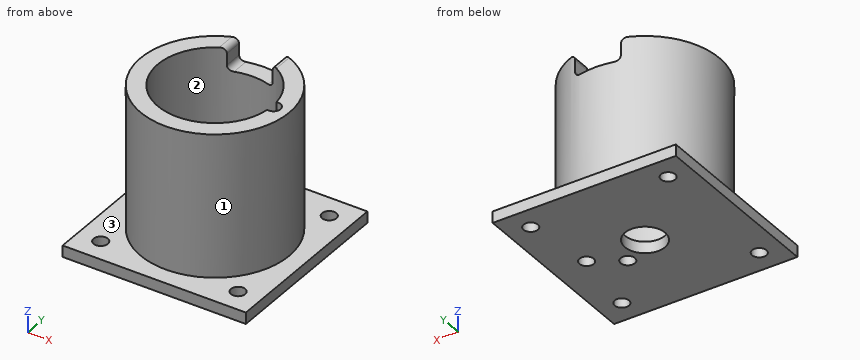
Autodesk Inventor part; units mm, degrees
ref_plane "Work Plane1" through (0, 16.51, 0) normal (0, 1, 0) x (-1, 0, 0)
ref_plane "YZ Plane" through (0, 0, 0) normal (1, 0, 0) x (0, 1, 0)
ref_plane "XY Plane" through (0, 0, 0) normal (0, 0, 1) x (1, 0, 0)
sketch "Sketch1" plane through (0, 0, 0) normal (0, 0, 1) x (1, 0, 0)
  line L0 (20.32, 20.32) -> (-20.32, 20.32)
  line L1 (-20.32, 20.32) -> (-20.32, -20.32)
  line L2 (-20.32, -20.32) -> (20.32, -20.32)
  line L3 (20.32, -20.32) -> (20.32, 20.32)
  point P0 (0, 0)
  dimension "d0" = 40.64
  dimension "d1" = 40.64
  dimension "d2" = 20.32
  dimension "d3" = 20.32
extrude "Extrusion1" add sketch "Sketch1" along normal blind 2.54
sketch "Sketch2" plane through (0, 0, 2.54) normal (0, 0, 1) x (1, 0, 0)
  circle A0 centre (0, 0) radius 12.7
  circle A1 centre (0, 0) radius 16.51
  dimension "d6" = 25.4
  dimension "d7" = 3.81
extrude "Extrusion2" add sketch "Sketch2" along normal blind 31.75
sketch "Sketch3" plane through (0, 0, 2.54) normal (0, 0, 1) x (1, 0, 0)
  line L0 (20.32, 20.32) -> (-20.32, 20.32)
  line L1 (-20.32, 20.32) -> (-20.32, -20.32)
  line L2 (20.32, -20.32) -> (20.32, 20.32)
  line L3 (-20.32, -20.32) -> (20.32, -20.32)
  point P0 (0, 0)
  point P1 (-15.24, -15.24)
  point P2 (15.24, -15.24)
  point P3 (15.24, 15.24)
  point P4 (-15.24, 15.24)
  dimension "d10" = 5.08
  dimension "d11" = 5.08
  dimension "d12" = 5.08
  dimension "d13" = 5.08
  dimension "d14" = 5.08
  dimension "d15" = 5.08
  dimension "d16" = 5.08
  dimension "d17" = 5.08
hole "Hole1" at (-15.24, -15.24, 2.54) at (15.24, -15.24, 2.54) at (15.24, 15.24, 2.54) at (-15.24, 15.24, 2.54) direction (0, 0, -1) diameter 3.175 depth 3.175 tip angle 118
ref_plane "Work Plane1" through (0, 16.51, 0) normal (0, 1, 0) x (-1, 0, 0)
sketch "Sketch4" plane through (0, 16.51, 0) normal (0, 1, 0) x (-1, 0, 0)
  line L0 (-12.7, 34.29) -> (12.7, 34.29)
  line L1 (5.08, 34.29) -> (-5.08, 34.29)
  line L2 (-5.08, 34.29) -> (-5.08, 29.21)
  line L3 (-5.08, 29.21) -> (5.08, 29.21)
  line L4 (5.08, 29.21) -> (5.08, 34.29)
  line L5 (0, -6.858) -> (0, 41.148)
  point P0 (0, 0)
  dimension "d26" = 5.08
  dimension "d27" = 10.16
  dimension "d28" = 5.08
extrude "Extrusion3" cut sketch "Sketch4" against normal blind 10.16
sketch "Sketch5" plane through (0, 0, 2.54) normal (0, 0, 1) x (1, 0, 0)
  circle A0 centre (0, 0) radius 4.445
  dimension "d31" = 8.89
extrude "Extrusion4" cut sketch "Sketch5" against normal through all
fillet "Fillet1" radius 1.27 4 edges at (-5.08, 13.6744, 29.21) (-5.08, 13.6744, 34.29) (5.08, 13.6744, 34.29) (5.08, 13.6744, 29.21)
sketch "Sketch6" plane through (0, 0, 0) normal (0, 0, -1) x (-1, 0, 0)
  circle A0 centre (-6.4775, -4.0132) radius 3.81 construction
  line L0 (20.32, -20.32) -> (-20.32, -20.32) construction
  circle A1 centre (0, 0) radius 3.81 construction
  circle A2 centre (-6.4775, -4.0132) radius 1.5875
  circle A3 centre (-12.9551, 0) radius 3.81 construction
  line L1 (20.32, 20.32) -> (20.32, -20.32)
  circle A4 centre (-12.9551, 0) radius 1.5875
  dimension "d35" = 16.3068
  dimension "d36" = 7.62
  dimension "d37" = 7.62
  dimension "d38" = 3.175
  dimension "d39" = 7.62
  dimension "d41" = 20.32
  dimension "d42" = 3.175
extrude "Extrusion5" cut sketch "Sketch6" against normal through all
properties part number "000114"
Input: part model. Units: mm. Frame: model coordinates. Face numbers are marked on the shaded views. Give positions to 0.01 mm unless a question says otherwise; leave off trailing zeros. Order: outer loops, then holes, each group sorted by start corner. A loop starts at its lowest first (then second) coordinate and runs counter-clockwise, first axis right, second up.
1. Mould query, pull axis X, two halves, no side actions, for the marked faces 1, 2 and 3. Classes: released by +X, released by -X, zero draft, split by the parting line, or undercut.
Derived:
face 1: split by the parting line
face 2: undercut
face 3: zero draft
2. Section C-C on x = 15.24. Return the cut outline in (y, z), and give its area (3 significant figures).
Derived:
outline: (-20.32, 0) - (-16.83, 0) - (-16.83, 2.54) - (-20.32, 2.54) - close; (-13.65, 0) - (13.65, 0) - (13.65, 2.54) - (6.35, 2.54) - (6.35, 34.29) - (-6.35, 34.29) - (-6.35, 2.54) - (-13.65, 2.54) - close; (16.83, 0) - (20.32, 0) - (20.32, 2.54) - (16.83, 2.54) - close
area: 490 mm2
3. Section D-D on y = -5. Return the cut outline in (x, z), and give its area (3 significant figures).
Derived:
outline: (-20.32, 0) - (5.23, 0) - (5.23, 2.54) - (-11.67, 2.54) - (-11.67, 34.29) - (-15.73, 34.29) - (-15.73, 2.54) - (-20.32, 2.54) - close; (7.72, 0) - (20.32, 0) - (20.32, 2.54) - (15.73, 2.54) - (15.73, 34.29) - (11.67, 34.29) - (11.67, 2.54) - (7.72, 2.54) - close
area: 355 mm2
4. Pin query (flat end, axial travel): pin 1 (0.8 mm diameter, centred on y = 13.5, z = 32, fed in from +X); pin 2 (3 mm diameter, centred on x = -16, z = 22.5, fed in from -Y); pin 3 (10 mm diameter, centred on x = 12.5, z = 20, fed in from -Y). Return the tip coordinate at first contact, or that it passes through.
Derived:
pin 1: stops at x = 10.05
pin 2: stops at y = -7.89
pin 3: stops at y = -14.71
5. Material intervals for L1, parallel to X at y = 15.24, z = 1.2; L2, parallel to X at y = 0, z = 15; L3, parallel to Y at x = 0, z = 17, sorted ascending.
Derived:
L1: x = -20.32 to -16.83, -13.65 to 13.65, 16.83 to 20.32
L2: x = -16.51 to -12.7, 14.54 to 16.51
L3: y = -16.51 to -12.7, 12.7 to 16.51
6. Section A-A on y = 0. Return the cut outline in (x, z) (3 decimals), and give its area (3 significant figures).
Derived:
outline: (-20.32, 0) - (-4.445, 0) - (-4.445, 2.54) - (-12.7, 2.54) - (-12.7, 34.29) - (-16.51, 34.29) - (-16.51, 2.54) - (-20.32, 2.54) - close; (4.445, 0) - (11.368, 0) - (11.368, 2.54) - (4.445, 2.54) - close; (14.543, 0) - (20.32, 0) - (20.32, 2.54) - (16.51, 2.54) - (16.51, 34.29) - (14.543, 34.29) - close
area: 256 mm2
7. Section B-B on x = 0. Return the cut outline in (y, z) (3 decimals).
Derived:
outline: (-20.32, 0) - (-4.445, 0) - (-4.445, 2.54) - (-12.7, 2.54) - (-12.7, 34.29) - (-16.51, 34.29) - (-16.51, 2.54) - (-20.32, 2.54) - close; (4.445, 0) - (20.32, 0) - (20.32, 2.54) - (16.51, 2.54) - (16.51, 29.21) - (12.7, 29.21) - (12.7, 2.54) - (4.445, 2.54) - close
